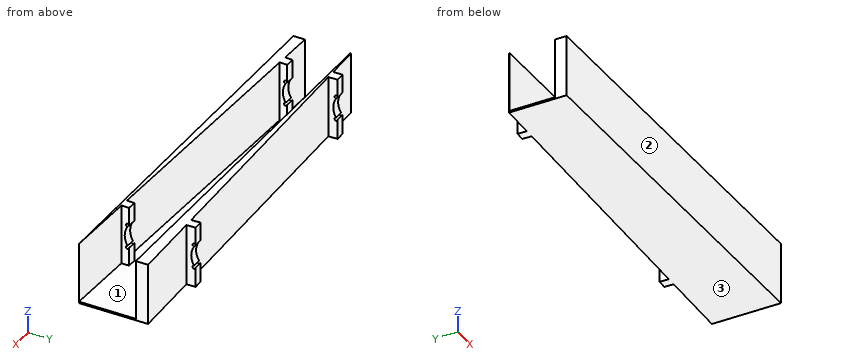
```python
from build123d import *

# Parameters (mm, degrees)
PAD_DEPTH       = 80
POCKET_DEPTH    = 78
POCKET001_DEPTH = 408.7079232475
POCKET002_DEPTH = 408.4326470939


with BuildPart() as part:
    # Sketch → Pad (new body)
    with BuildSketch(Plane.XY):
        Polygon((450, 0), (450, 90), (356, 87.18), (355.64, 99.18), (343.64, 98.82), (344, 86.82), (6, 76.68), (5.64, 88.6800000001), (-6.36, 88.3200000001), (-6, 76.32), (-50, 75), (-50, 0), align=None)
    extrude(amount=PAD_DEPTH)

    # Sketch001 (on Face14 of Pad) → Pocket (cut)
    with BuildSketch(Plane.XY.offset(80)):
        Polygon((-50, 15), (-50, 74), (450, 74), (450, 0), (356, 2.82), (356.3, 12.82), (344.3, 13.18), (344, 3.18), (6, 13.32), (6.3, 23.32), (-5.7, 23.68), (-6, 13.68), align=None)
    extrude(amount=-POCKET_DEPTH, mode=Mode.SUBTRACT)

    # Sketch002 (on Face26 of Pocket) → Pocket001 (cut, through all)
    with BuildSketch(Plane(origin=(355.5953641722, -10.6678609252, 0), x_dir=(0.0299865091, 0.9995503035, 0), z_dir=(0.9995503035, -0.0299865091, 0))):
        with BuildLine():
            ThreePointArc((23.4984280855, 56), (19.9988591841, 57.4495689014), (21.4484280855, 53.95))
            ThreePointArc((21.4484280855, 53.95), (17.8329435114, 41), (21.4484280855, 28.05))
            ThreePointArc((21.4484280855, 28.05), (19.9988591841, 24.5504310986), (23.4984280855, 26))
            Line((23.4984280855, 26), (23.4984280855, 56))
        make_face()
    extrude(amount=-POCKET001_DEPTH, mode=Mode.SUBTRACT)

    # Sketch003 (on Face14 of Pocket001) → Pocket002 (cut, through all)
    with BuildSketch(Plane(origin=(358.2929363573, 10.7487880907, 0), x_dir=(-0.0299865091, 0.9995503035, 0), z_dir=(0.9995503035, 0.0299865091, 0))):
        with BuildLine():
            ThreePointArc((88.470997005, 56), (84.9714281036, 57.4495689014), (86.420997005, 53.95))
            ThreePointArc((86.420997005, 53.95), (82.8055124309, 41), (86.420997005, 28.05))
            ThreePointArc((86.420997005, 28.05), (84.9714281036, 24.5504310986), (88.470997005, 26))
            Line((88.470997005, 26), (88.470997005, 56))
        make_face()
    extrude(amount=-POCKET002_DEPTH, mode=Mode.SUBTRACT)


solid = part.part
```
For this review, take the finished solid that the model builds, in its own axes (mm). Face numbers are marked on the shaded views. Give positions to 0.01 mm unless a question says otherwise; leave off trailing zeros. Loops run counter-clockwise (first coordinate to the right, second up) from the corner with the lowest first, then second, coordinate; pieces in that order, holes last. Notation, with made-up numbers: M 2,8 L 49,8 A22 ccw 49,45 Z; hole C -6,-3.75 d8. An arc over 180 degrees is marked long. One line per item, written item: value. Start each with the question number.
Q1. Add section C-C (y = 48.5). Give the boundary of the cut face in (x, z), and give its area (3 significant figures).
Q2. Clearance check with flat-ended pins moving along their axes: pin 1 Ø1 at (x, y) = (315.5, 51) entering from -Z; pin 2 Ø3 at (y, z) = (80, 59) entering from -X. State where each tip first meets the part, or that it passes through.
Q3. Add section B-B (x = 239). Give the boundary of the cut face in (y, z).
Q4. Add section D-D (x = 396). Give the boundary of the cut face in (y, z), and give its area (3 significant figures).
Q5. Add section A-A (z = 7.5). Give the boundary of the cut face in (x, y).
Q6. Draft analysis for pull direction Y (two halves, no side actions). For the marked faces 1, 2 and 3, state which applies: released by +Y, released by -Y, zero draft, split by the parting line, or undercut.
Q7. For L1, parallel to Z at x = -23.5, y = 28; L2, parallel to X at y = 22.5, z = 65; L3, parallel to Y at x = -1, z = 20.5, list the stretches that pass through material, from the lowest coordinate up.
Reply:
1. outline: M -50,0 L 450,0 L 450,2 L -50,2 Z
1. area: 1,000 mm²
2. pin 1: z = 0
2. pin 2: x = -6.16
3. outline: M 0,0 L 83.67,0 L 83.67,80 L 74,80 L 74,2 L 6.33,2 L 6.33,80 L 0,80 Z
4. outline: M 0,0 L 88.38,0 L 88.38,80 L 74,80 L 74,2 L 1.62,2 L 1.62,80 L 0,80 Z
4. area: 1,420 mm²
5. outline: M -50,0 L 450,0 L 356,2.82 L 356.3,12.82 L 344.3,13.18 L 344,3.18 L 6,13.32 L 6.3,23.32 L -5.7,23.68 L -6,13.68 L -50,15 Z; M -50,74 L 450,74 L 450,90 L 356,87.18 L 355.64,99.18 L 343.64,98.82 L 344,86.82 L 6,76.68 L 5.64,88.68 L -6.36,88.32 L -6,76.32 L -50,75 Z
6. face 1: undercut
6. face 2: released by -Y
6. face 3: zero draft
7. L1: 0 to 2
7. L2: -5.74 to 6.28
7. L3: 0 to 23.54, 74 to 88.48
